```python
from build123d import *

# Parameters (mm, degrees)
CUT_EXTRUDE1_DEPTH              = 161.078105936
M8X1_0_TAPPED_HOLE2_D           = 7
M8X1_0_TAPPED_HOLE2_DEPTH       = 21
M8X1_0_TAPPED_HOLE2_CSINK_D     = 8.05
M8X1_0_TAPPED_HOLE2_CSINK_ANGLE = 90
M8X1_0_TAPPED_HOLE2_TIP         = 2.103012167


with BuildPart() as part:
    # Sketch2 → Revolve1 (revolve)
    with BuildSketch(Plane.XY, mode=Mode.PRIVATE) as revolve1_sk:
        Polygon((55, 0), (100, 45), (100, 75), (88, 75), (88, 49.970562748), (50.029437252, 12), (0, 12), (0, 0), align=None)
    revolve(revolve1_sk.sketch.rotate(Axis((0, 0, 0), (0, 1, 0)), 90), axis=Axis((0, 0, 0), (0, 1, 0)))

    # Sketch3 → Cut-Extrude1 (cut, through all)
    with BuildSketch(Plane.XZ):
        with BuildLine():
            Line((-15, 18.5), (15, 18.5))
            ThreePointArc((15, 18.5), (21, 12.5), (15, 6.5))
            Line((15, 6.5), (-15, 6.5))
            ThreePointArc((-15, 6.5), (-21, 12.5), (-15, 18.5))
        make_face()
        with BuildLine():
            Line((-15, -6.5), (15, -6.5))
            ThreePointArc((15, -6.5), (21, -12.5), (15, -18.5))
            Line((15, -18.5), (-15, -18.5))
            ThreePointArc((-15, -18.5), (-21, -12.5), (-15, -6.5))
        make_face()
    extrude(amount=-CUT_EXTRUDE1_DEPTH, mode=Mode.SUBTRACT)

    # M8x1.0 Tapped Hole2
    with Locations(Plane(origin=(0, 75, 0), x_dir=(1, 0, 0), z_dir=(0, 1, 0))):
        with Locations((0, 94), (58.139395742, 73.863459591), (93.340114142, 11.118592175), (66.468037432, -66.468037432), (0, -94), (-66.468037432, -66.468037432), (-94, 0), (-66.468037432, 66.468037432)):
            CounterSinkHole(M8X1_0_TAPPED_HOLE2_D / 2, M8X1_0_TAPPED_HOLE2_CSINK_D / 2, depth=M8X1_0_TAPPED_HOLE2_DEPTH, counter_sink_angle=M8X1_0_TAPPED_HOLE2_CSINK_ANGLE)
            with Locations((0, 0, -(M8X1_0_TAPPED_HOLE2_DEPTH + M8X1_0_TAPPED_HOLE2_TIP / 2))):  # 118° drill point
                Cone(0, M8X1_0_TAPPED_HOLE2_D / 2, M8X1_0_TAPPED_HOLE2_TIP, mode=Mode.SUBTRACT)


solid = part.part
```
Model file for the job. Use its own axes, mm. A direction names the side the tool comes from. Coordinates: 2 decimals unless noted, no trailing zeros. Write each loop counter-clockwise with the first axis right and the second up, starting at its lowest first coordinate (ties: lowest second). Pieces come first, ordered by that corner, then holes. Notation, with made-up numbers: (36.5, 18.25) - (77.5, 18.25) arc R21 cw to (77.5, 42.25) - close; hole circle Ø7 at (-19.75, -20). An arc over 180 degrees is marked (long way). One line per question, with ' | ' between items. Start each with the question number.
Q1. 3-axis set-ups, long thin cutter, end or side, ignore diameter. For faces 4 (the face through (-1, 12, 1)), 5 (the face through (21, 5.9, -12.4)): which of +Z, -Z, +X, -X, +Y, -Y reach the whole face in a straight line?
Q2. Cut at A-A, the plane y = 35. List the corners of the cut face in (x, z).
Q3. Drill centre lines: line 1 (Z direction, x = -13, y = 49.5); line 2 (Z direction, x = -36, y = 38.5); line 3 (X direction, y = 41.5, z = 42.5). Where is each one in solid material? Low to high. Write a range as [from, to].
Q4. Cut at B-B, the plane x = -11. Give the number of separate pieces and of enclosed holes in the cut face, then the cut area to 3 significant figures.
Q5. Pull direction X, two halves, no side cores. Call faces 1 (the face through (59, 75, -66)), 2 (the face through (-66.916, 52.262, 66.057)), 3 (the face through (51.292, 2.815, -26.678)): pulls with the +X half, pulls with the -X half, needs draft (parallel to the pull), parting line crosses it, or undercut.
Q6. Pin check, flat tips, straight feed: pin 1 (4 mm diameter, centred on x = 0, z = 94, fed in from +Y); pin 2 (6 mm diameter, centred on y = 52.5, z = 50.5, fed in from +X); pin 3 (5 mm diameter, centred on y = 57.5, z = -8.5, fed in from -X); pin 4 (2 mm diameter, centred on x = 77.5, z = 66, fed in from +Y). Stop position of each tip, or through.
Answer below:
1) face 4: +Y | face 5: +Y, -Y
2) outline: circle Ø180 at (0, 0); hole circle Ø146.06 at (0, 0)
3) line 1: [-99.15, -86.56], [86.56, 99.15] | line 2: [-86.29, -67.53], [67.53, 86.29] | line 3: [-86.64, -67.22], [67.22, 86.64]
4) separate pieces: 3 | enclosed holes: 0 | area: 3,030 mm^2
5) face 1: needs draft | face 2: undercut | face 3: parting line crosses it
6) pin 1: y = 53.1 | pin 2: x = 88 | pin 3: x = -99.82 | pin 4: through
